Can you work these out from the model? Positions are in its coordinate system, mm. A direction names the side the tool comes from. Coordinates: 2 decimals unless noted, no trailing zeros. Write each loop counter-clockwise with the first axis right and the second up, starting at its lowest first coordinate (ties: lowest second). Pieces come first, ordered by that corner, then holes. Notation, with made-up numbers: (-19, 0.25) -> (25, 0.25) arc R15 cw to (25, 14.25) -> close; hole circle Ø5 at (20.5, 9.25). An arc over 180 degrees is marked (long way). Use one line per item in the form item = value.
```python
from build123d import *

# Parameters (mm, degrees)
BOSS_EXTRUDE1_DEPTH = 45
BOSS_EXTRUDE1_DRAFT = -20
BOSS_EXTRUDE3_DEPTH = 25
BOSS_EXTRUDE4_DEPTH = 66.34
BOSS_EXTRUDE4_TAPER = 20
SKETCH5_W           = 60
SKETCH5_H           = 136.34
CUT_EXTRUDE4_DEPTH  = 15
CIRPATTERN1_COUNT   = 6
SHELL1_T            = -5
SKETCH6_W           = 15
SKETCH6_H           = 26
CUT_EXTRUDE5_DEPTH  = 10


with BuildPart() as part:
    # Sketch1 → Boss-Extrude1 (with draft: the straight prism first)
    with BuildSketch(Plane.XY):
        Polygon((0, 57.15767665), (-49.5, 28.578838325), (-49.5, -28.578838325), (0, -57.15767665), (49.5, -28.578838325), (49.5, 28.578838325), align=None)
    extrude(amount=BOSS_EXTRUDE1_DEPTH)
    # Boss-Extrude1: the draft: its side faces are tilted about the plane it starts from
    boss_extrude1_sides = [part.faces().sort_by_distance(p)[0] for p in [
        (-24.75, 42.868257487, 22.5),
        (-49.5, 0, 22.5),
        (-24.75, -42.868257487, 22.5),
        (24.75, -42.868257487, 22.5),
        (49.5, 0, 22.5),
        (24.75, 42.868257487, 22.5),
    ]]
    draft(boss_extrude1_sides, Plane.XY, BOSS_EXTRUDE1_DRAFT)

    # Sketch3 → Boss-Extrude3 (add)
    with BuildSketch(Plane.XY.offset(45)):
        Polygon((0, -76.070124796), (65.878660542, -38.035062398), (65.878660542, 38.035062398), (0, 76.070124796), (-65.878660542, 38.035062398), (-65.878660542, -38.035062398), align=None)
    extrude(amount=BOSS_EXTRUDE3_DEPTH)

    # Sketch4 → Boss-Extrude4 (add)
    with BuildSketch(Plane.XY.offset(70)):
        Polygon((65.878660542, -38.035062398), (65.878660542, 38.035062398), (0, 76.070124796), (-65.878660542, 38.035062398), (-65.878660542, -38.035062398), (0, -76.070124796), align=None)
    extrude(amount=BOSS_EXTRUDE4_DEPTH, taper=BOSS_EXTRUDE4_TAPER)

    # Sketch5 → Cut-Extrude4 (cut)
    with BuildSketch(Plane(origin=(0, 77, 0), x_dir=(1, 0, 0), z_dir=(0, 1, 0))):
        with Locations((0, -68.17)):
            Rectangle(SKETCH5_W, SKETCH5_H)
    cut_extrude4 = extrude(amount=-CUT_EXTRUDE4_DEPTH, mode=Mode.SUBTRACT)

    # CirPattern1: Cut-Extrude4 ×6 about axis
    cirpattern1_axis = Axis((0, 0, 0), (0, 0, 1))
    for i in range(1, CIRPATTERN1_COUNT):
        add(cut_extrude4.rotate(cirpattern1_axis, i * 360 / CIRPATTERN1_COUNT), mode=Mode.SUBTRACT)

    # Shell1
    shell1_openings = [part.faces().sort_by_distance(p)[0] for p in [
        (0, 0, 0),
    ]]
    offset(amount=SHELL1_T, openings=shell1_openings, kind=Kind.INTERSECTION)

    # Sketch6 → Cut-Extrude5 (cut)
    with BuildSketch(Plane(origin=(32.939330271, 57.052593597, 0), x_dir=(0.8660254037844417, -0.49999999999999467, 0), z_dir=(0.49999999999999467, 0.8660254037844417, 0))):
        with Locations((0.105187193, -57.5)):
            Rectangle(SKETCH6_W, SKETCH6_H)
    extrude(amount=-CUT_EXTRUDE5_DEPTH, mode=Mode.SUBTRACT)


solid = part.part
```
Q1. Will these pins go through, and if not, where does the flat tip stop? pin 1 (3 mm diameter, centred on x = 37, z = 96.5, fed in from +Y); pin 2 (5 mm diameter, centred on y = -38.5, z = 87.5, fed in from -X); pin 3 (3 mm diameter, centred on x = -28, y = 0.5, fed in from -Z).
Return value:
pin_1 = 44.64
pin_2 = -50.81
pin_3 = 131.34
Q2. If I drill on line 1 (Y direction, x = -20.5, z = 64.5); line 2 (Y direction, x = -20.5, z = 81); line 3 (X direction, y = 16, z = 24), over which ranges is the centre line in solid material (lowest first)? Write a range as from..to.
Return value:
line_1 = -62..-57, 57..62
line_2 = -59.61..-53.47, 53.47..59.61
line_3 = -58.24..-52.91, 52.91..58.24
Q3. Suppose I cut it at C-C (x = 12). Write out the boundary of the cut face in (y, z).
Return value:
outline = (-62, 28.01) -> (-50.23, 0) -> (-44.09, 0) -> (-57, 30.73) -> (-57, 84.27) -> (-37.22, 131.34) -> (37.22, 131.34) -> (57, 84.27) -> (57, 30.73) -> (44.09, 0) -> (50.23, 0) -> (62, 28.01) -> (62, 86.99) -> (41.26, 136.34) -> (-41.26, 136.34) -> (-62, 86.99) -> close
Q4. Thinking about a two-plate mould opening in Y: for faces 4 (the flat face through (-26.61, -46.96, 102.71)), 5 (the flat face through (53.52, 31.3, 56.86)), 6 (the flat face through (49.714, 0.399, 99.794)), which applies, released by +Y, released by -Y, zero draft, split by the parting line, or undercut?
Return value:
face_4 = released by -Y
face_5 = released by +Y
face_6 = undercut
Q5. Suppose I cut it at D-D (z = 29). Write out the boundary of the cut face in (x, y), then the cut area to 3 significant figures.
Return value:
outline = (-60.06, -19.98) -> (-47.33, -42.02) -> (-12.72, -62) -> (12.72, -62) -> (47.33, -42.02) -> (60.06, -19.98) -> (60.06, 19.98) -> (47.33, 42.02) -> (12.72, 62) -> (-12.72, 62) -> (-47.33, 42.02) -> (-60.06, 19.98) -> close; hole (-54.73, -19.2) -> (-43.99, -37.8) -> (-10.74, -57) -> (10.74, -57) -> (43.99, -37.8) -> (54.73, -19.2) -> (54.73, 19.2) -> (43.99, 37.8) -> (10.74, 57) -> (-10.74, 57) -> (-43.99, 37.8) -> (-54.73, 19.2) -> close
area = 1,950 mm2
Q6. Suppose I cut it at A-A (z = 92.5). Write out the boundary of the cut face in (x, y), then the cut area to 3 significant figures.
Return value:
outline = (-57.69, -24.08) -> (-49.7, -37.92) -> (-7.99, -62) -> (7.99, -62) -> (49.7, -37.92) -> (57.69, -24.08) -> (57.69, 24.08) -> (49.7, 37.92) -> (7.99, 62) -> (-7.99, 62) -> (-49.7, 37.92) -> (-57.69, 24.08) -> close; hole (-52.37, -23.3) -> (-46.36, -33.7) -> (-6.01, -57) -> (6.01, -57) -> (46.36, -33.7) -> (52.37, -23.3) -> (52.37, 23.3) -> (46.36, 33.7) -> (6.01, 57) -> (-6.01, 57) -> (-46.36, 33.7) -> (-52.37, 23.3) -> close
area = 1,930 mm2
Q7. Suppose I cut it at B-B (y = -2.5). Write out the boundary of the cut face in (x, z), then the cut area to 3 significant figures.
Return value:
outline = (-65.88, 45) -> (-49.5, 0) -> (-44.18, 0) -> (-60.88, 45.88) -> (-60.88, 69.12) -> (-38.23, 131.34) -> (38.23, 131.34) -> (60.88, 69.12) -> (60.88, 45.88) -> (44.18, 0) -> (49.5, 0) -> (65.88, 45) -> (65.88, 70) -> (41.73, 136.34) -> (-41.73, 136.34) -> (-65.88, 70) -> close
area = 1,810 mm2
Q8. For faces 1 (the flat face through (24.511, 43.253, 99.794)), 2 (the flat face through (25.18, 58.4, 57.68)), 3 (the flat face through (-32.82, 57.12, 57.32)), which set-ups out of +Z, -Z, +X, -X, +Y, -Y let a thin tool reach every point of the face, with its end or its side?
Return value:
face_1 = none
face_2 = +X
face_3 = +Z, -Z, -X, +Y
